Autodesk Fusion 360 part; units mm, degrees
sketch "草图1" plane through (0, 0, 0) normal (0, 0, 1) x (1, 0, 0)
  line L0 (28.4627, -32.3648) -> (28.4702, -32.3737)
  line L1 (41.5939, -11.2943) -> (41.768, -11.325)
  arc A0 (14.7507, -46.3074) -> (13.8402, -43.4489) centre (14.2954, -44.8782) ccw construction
  line L2 (-28.4627, -32.3648) -> (-28.4702, -32.3737)
  circle A1 centre (0, -47.1) radius 1.4
  line L3 (43.1, 0) -> (48, 0) construction
  line L4 (0, -43.1) -> (0, -51.1) construction
  arc A2 (2.5554, -45.5283) -> (2.6381, -48.5283) centre (0, -47.1) ccw construction
  circle A3 centre (0, 0) radius 44.72 construction
  arc A4 (2.6381, -48.5283) -> (14.7507, -46.3074) centre (0, 0) ccw construction
  line L5 (-30.5781, -30.3742) -> (-30.6917, -30.5096)
  line L6 (-41.5939, -11.2943) -> (-41.768, -11.325)
  line L7 (30.5781, -30.3742) -> (30.6917, -30.5096)
  line L8 (42.2601, -8.467) -> (42.2716, -8.469)
  line L9 (-42.2601, -8.467) -> (-42.2716, -8.469)
  line L10 (0.9, -43.0906) -> (0.9, -43.1)
  arc A5 (2.5554, -45.5283) -> (13.8402, -43.4489) centre (0, 0) ccw construction
  line L11 (-0.9, -43.0906) -> (-0.9, -43.1)
  circle A6 centre (0, 0) radius 43.1
  arc A7 (40.7077, 26.5489) -> (32.728, 35.9282) centre (0, 0) ccw construction
  line L12 (11.0158, 41.6685) -> (11.0763, 41.8346)
  line L13 (13.7974, 40.8319) -> (13.8014, 40.8428)
  line L14 (36.8676, 22.3247) -> (36.8757, 22.3294)
  arc A8 (32.728, 35.9282) -> (30.7078, 33.7104) centre (31.7179, 34.8193) ccw construction
  circle A9 centre (40.7898, 23.55) radius 1.4
  circle A10 centre (-40.7898, 23.55) radius 1.4
  line L15 (-15.6751, 9.05) -> (-16.3679, 9.45) construction
  arc A11 (38.151, 24.9772) -> (30.7078, 33.7104) centre (0, 0) ccw construction
  line L16 (-13.7974, 40.8319) -> (-13.8014, 40.8428)
  line L17 (37.7676, 20.7659) -> (37.7757, 20.7706)
  arc A12 (-40.7064, 20.5512) -> (-44.548, 9.7385) centre (0, 0) ccw construction
  arc A13 (-47.4788, 10.3792) -> (-44.548, 9.7385) centre (-46.0134, 10.0589) ccw construction
  circle A14 centre (0, 0) radius 47.1 construction
  arc A15 (-43.3459, 21.9795) -> (-47.4788, 10.3792) centre (0, 0) ccw construction
  line L18 (-37.7676, 20.7659) -> (-37.7757, 20.7706)
  line L19 (-36.8676, 22.3247) -> (-36.8757, 22.3294)
  arc A16 (38.151, 24.9772) -> (40.7077, 26.5489) centre (40.7898, 23.55) ccw construction
  circle A17 centre (0, 0) radius 47.1 construction
  line L20 (-11.0158, 41.6685) -> (-11.0763, 41.8346)
  line L21 (-37.3257, 21.55) -> (-41.5692, 24) construction
  arc A18 (-40.7064, 20.5512) -> (-43.3459, 21.9795) centre (-40.7898, 23.55) ccw construction
  circle A19 centre (0, 0) radius 46.9
  arc A20 (32.5934, 35.7803) -> (30.8425, 33.8583) centre (31.7179, 34.8193) ccw
  arc A21 (38.3851, 24.9844) -> (30.8425, 33.8583) centre (0, 0) ccw
  arc A22 (38.3851, 24.9844) -> (40.6026, 26.3437) centre (40.7898, 23.55) ccw
  arc A23 (40.6026, 26.3437) -> (32.5934, 35.7803) centre (0, 0) ccw
  arc A24 (2.4446, -45.7347) -> (13.9009, -43.6395) centre (0, 0) ccw
  arc A25 (14.69, -46.1168) -> (13.9009, -43.6395) centre (14.2954, -44.8782) ccw
  arc A26 (2.5131, -48.3347) -> (14.69, -46.1168) centre (0, 0) ccw
  arc A27 (2.4446, -45.7347) -> (2.5131, -48.3347) centre (0, -47.1) ccw
  arc A28 (-47.2834, 10.3365) -> (-44.7434, 9.7812) centre (-46.0134, 10.0589) ccw
  arc A29 (-40.8297, 20.7503) -> (-44.7434, 9.7812) centre (0, 0) ccw
  arc A30 (-40.8297, 20.7503) -> (-43.1156, 21.991) centre (-40.7898, 23.55) ccw
  arc A31 (-43.1156, 21.991) -> (-47.2834, 10.3365) centre (0, 0) ccw
  circle A32 centre (0, 0) radius 19.5
  dimension "d43" = 1.8
  dimension "d44" = 6
  dimension "d45" = 3
  dimension "d46" = 2.8
  dimension "d47" = 2.8
  dimension "d48" = 2.8
  dimension "d49" = 86.2
  dimension "d53" = -0.2
  dimension "d54" = -0.2
  dimension "d55" = -0.2
  dimension "d56" = -0.2
  dimension "d57" = 39
extrude "拉伸5" add sketch "草图1" along normal blind 1.8 contours A1 A19 A25 A26 A27 | A1 A19 A24 A25 A27 | A19 A20 A21 A22 A24 A25 A27 A28 A29 A30 | A10 A19 A28 A30 A31 | A10 A19 A28 A29 A30 | A9 A19 A20 A21 A22 | A9 A19 A20 A22 A23
extrude "拉伸6" add sketch "草图1" along normal up to surface (1.8 mm away) contours A6
sketch "草图3" plane through (0, 0, 1.8) normal (0, 0, 1) x (-1, 0, 0)
  circle A0 centre (0, 0) radius 19.5
  circle A1 centre (40.7898, -23.55) radius 1.4
  circle A2 centre (-40.7898, -23.55) radius 1.4
  circle A3 centre (0, 47.1) radius 1.4
  arc A4 (43.1156, -21.991) -> (47.2834, -10.3365) centre (0, 0) ccw
  arc A5 (47.2834, -10.3365) -> (46.0746, -8.7603) centre (46.0134, -10.0589) ccw
  arc A6 (46.0746, -8.7603) -> (2.7857, 46.8172) centre (0, 0) ccw
  arc A7 (2.7857, 46.8172) -> (-2.5131, 48.3347) centre (0, 47.1) ccw
  arc A8 (-2.5131, 48.3347) -> (-14.69, 46.1168) centre (0, 0) ccw
  arc A9 (-14.69, 46.1168) -> (-15.4506, 44.2819) centre (-14.2954, 44.8782) ccw
  arc A10 (-15.4506, 44.2819) -> (-41.9377, -20.9961) centre (0, 0) ccw
  arc A11 (-41.9377, -20.9961) -> (-40.6026, -26.3437) centre (-40.7898, -23.55) ccw
  arc A12 (-40.6026, -26.3437) -> (-32.5934, -35.7803) centre (0, 0) ccw
  arc A13 (-32.5934, -35.7803) -> (-30.6239, -35.5216) centre (-31.7179, -34.8193) ccw
  arc A14 (-30.6239, -35.5216) -> (39.152, -25.8211) centre (0, 0) ccw
  arc A15 (39.152, -25.8211) -> (43.1156, -21.991) centre (40.7898, -23.55) ccw
  circle A16 centre (0, 0) radius 29.75
  dimension "d64" = 59.5
sketch "草图4" plane through (0, 0, 0) normal (0, 0, -1) x (1, 0, 0)
  circle A0 centre (0, 0) radius 19.5
  circle A1 centre (-40.7898, -23.55) radius 1.4
  circle A2 centre (40.7898, -23.55) radius 1.4
  circle A3 centre (0, 47.1) radius 1.4
  arc A4 (-47.2834, -10.3365) -> (-43.1156, -21.991) centre (0, 0) ccw
  arc A5 (-43.1156, -21.991) -> (-39.152, -25.8211) centre (-40.7898, -23.55) ccw
  arc A6 (-39.152, -25.8211) -> (30.6239, -35.5216) centre (0, 0) ccw
  arc A7 (30.6239, -35.5216) -> (32.5934, -35.7803) centre (31.7179, -34.8193) ccw
  arc A8 (32.5934, -35.7803) -> (40.6026, -26.3437) centre (0, 0) ccw
  arc A9 (40.6026, -26.3437) -> (41.9377, -20.9961) centre (40.7898, -23.55) ccw
  arc A10 (41.9377, -20.9961) -> (15.4506, 44.2819) centre (0, 0) ccw
  arc A11 (15.4506, 44.2819) -> (14.69, 46.1168) centre (14.2954, 44.8782) ccw
  arc A12 (14.69, 46.1168) -> (2.5131, 48.3347) centre (0, 0) ccw
  arc A13 (2.5131, 48.3347) -> (-2.7857, 46.8172) centre (0, 47.1) ccw
  arc A14 (-2.7857, 46.8172) -> (-46.0746, -8.7603) centre (0, 0) ccw
  arc A15 (-46.0746, -8.7603) -> (-47.2834, -10.3365) centre (-46.0134, -10.0589) ccw
  circle A16 centre (0, 0) radius 43.1
  dimension "d65" = 86.2
extrude "拉伸8" add sketch "草图4" along normal blind 18 contours A16
extrude "拉伸9" cut sketch "草图3" against normal blind 5.5 contours A16
sketch "草图5" plane through (0, 0, -3.7) normal (0, 0, 1) x (-1, 0, 0)
  circle A0 centre (0, 0) radius 19.5
  circle A1 centre (0, 0) radius 29.75
  line L0 (0.0358, 19.5) -> (0.0358, 29.75)
  line L1 (8.0358, 17.7673) -> (8.0358, 28.6442)
  line L2 (-7.9642, 17.7673) -> (-7.9642, 28.6642)
extrude "拉伸10" cut sketch "草图5" against normal blind 20 contours A0 A1 L0 L1 | A0 A1 L0 L2
sketch "草图6" plane through (0, 0, -18) normal (0, 0, -1) x (1, 0, 0)
  circle A0 centre (0, 0) radius 43.1
  line L0 (-8.0358, 17.7673) -> (-8.0358, 28.6442)
  arc A1 (7.9642, 28.6642) -> (-8.0358, 28.6442) centre (0, 0) ccw
  line L1 (7.9642, 28.6642) -> (7.9642, 17.7995)
  arc A2 (-8.0358, 17.7673) -> (7.9642, 17.7995) centre (0, 0) ccw
  circle A3 centre (0, 0) radius 35
  circle A4 centre (0, -35) radius 1.31
  circle A5 centre (35, 0) radius 1.31
  circle A6 centre (0, 35) radius 1.31
  circle A7 centre (-35, 0) radius 1.31
  dimension "d73" = 70
  dimension "d74" = 2.62
  dimension "d76" = 360
extrude "拉伸11" cut sketch "草图6" against normal blind 8 contours A3 A5 | A3 A5 | A3 A6 | A3 A6 | A3 A4 | A3 A4 | A3 A7 | A3 A7
sketch "草图7" plane through (0, 0, -18) normal (0, 0, -1) x (1, 0, 0)
  circle A0 centre (35, 0) radius 1.31
  circle A1 centre (-35, 0) radius 1.31
  circle A2 centre (0, -35) radius 1.31
  circle A3 centre (0, 35) radius 1.31
  circle A4 centre (0, 0) radius 43.1
  line L0 (-8.0358, 17.7673) -> (-8.0358, 28.6442)
  arc A5 (7.9642, 28.6642) -> (-8.0358, 28.6442) centre (0, 0) ccw
  line L1 (7.9642, 28.6642) -> (7.9642, 17.7995)
  arc A6 (-8.0358, 17.7673) -> (7.9642, 17.7995) centre (0, 0) ccw
  circle A7 centre (0, 0) radius 30
  dimension "d79" = 60
extrude "拉伸12" cut sketch "草图7" against normal blind 10 contours A7
extrude "拉伸13" add 1 faces at (34.9911, 7.617, -18) along direction (0, 0, -1) blind 6
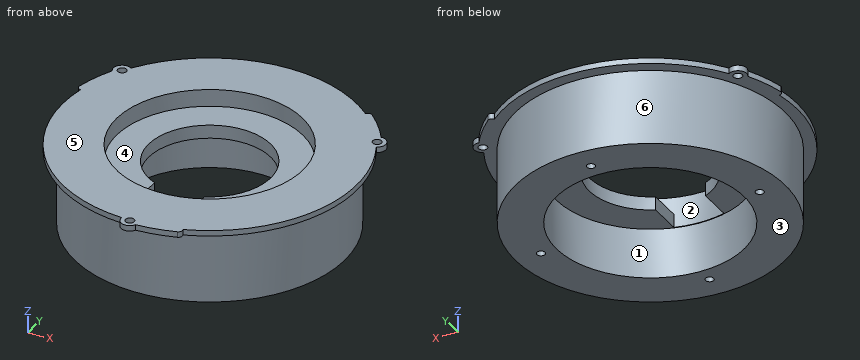
Here's how the part is built. I have some questions about the finished solid (model axes, mm). Face numbers are marked on the shaded views. A direction names the side the tool comes from. Give positions to 0.01 mm unless a question says otherwise; leave off trailing zeros. Order: outer loops, then holes, each group sorted by start corner. A loop starts at its lowest first (then second) coordinate and runs counter-clockwise, first axis right, second up. Notation, with made-up numbers: M 2.25,48 L 15.25,48 A26 ccw 15.25,62 Z; hole C -25,11.25 d9. An arc over 180 degrees is marked long. Use a Markdown table: item, result. Add a question column.
1. Suppose I cut it at A-A (x = 0). Give the number of separate pieces and of enclosed holes in the cut face, and give its area (3 significant figures).
2. For pin 1 Ø3 at (x, z) = (20.5, -2) entering from -Y; pin 2 Ø2 at (x, z) = (-25, -17) entering from -Y; pin 3 Ø4 at (x, z) = (-15, -16.5) entering from -Y, each with a flat end and sliding along its axis, tell me the tip position at first contact or that it passes through.
3. If we mould it in two halves opening along X, with no side actions, what happens to the marked faces 4, 5 and 6? For each: +X half, -X half, draft (parallel to the pull), parting line (faces both ways), or undercut.
4. Suppose I cut it at D-D (y = 23.55). List the corners of the cut face in (x, z) for me.
5. Suppose I cut it at C-C (z = -14.75). List the corners of the cut face in (x, y) for me, and give its area (3 significant figures).
6. I need wall thicknesses on probe 1 along X at (y, z) = (0, -5); probe 2 along X at (y, z) = (0, -14.5); probe 3 along Y at (x, z) = (0.5, -0.5). Which ranges of each line are inside material? Lowest first, please. Write a range as from..to.
7. Suppose I cut it at B-B (y = 0). List the corners of the cut face in (x, z) for me, and give its area (3 significant figures).
8. On a 3-axis mill with a long thin cutter (end or side, diameter ignored), from which of +Z, -Z, +X, -X, +Y, -Y can I reach the whole of each face in a straight line? I mean the marked faces 1, 2 and 3. Say none if no direction works.
Results list:
| question | item | result |
|---|---|---|
| 1 | separate pieces | 3 |
| 1 | enclosed holes | 0 |
| 1 | area | 666 mm² |
| 2 | pin 1 | stops at y = -38.69 |
| 2 | pin 2 | stops at y = -35.8 |
| 2 | pin 3 | stops at y = -41.09 |
| 3 | face 4 | undercut |
| 3 | face 5 | draft |
| 3 | face 6 | parting line |
| 4 | outline | M -43.59,0 L -42.19,0 L -42.19,1.8 L -43.59,1.8 Z; M -39.39,0 L -36.1,0 L -36.1,-24 L -18.58,-24 L -18.58,-8 L 18.58,-8 L 18.58,-24 L 36.1,-24 L 36.1,0 L 39.39,0 L 39.39,1.8 L 18.18,1.8 L 18.18,-3.7 L -18.18,-3.7 L -18.18,1.8 L -39.39,1.8 Z; M 42.19,0 L 43.59,0 L 43.59,1.8 L 42.19,1.8 Z |
| 5 | outline | C 0,0 d86.2; hole C -35,0 d2.62; hole C 0,0 d60; hole C 0,-35 d2.62; hole C 0,35 d2.62; hole C 35,0 d2.62 |
| 5 | area | 2,990 mm² |
| 6 | probe 1 | x = -43.1..-19.5, 19.5..43.1 |
| 6 | probe 2 | x = -43.1..-36.31, -33.69..-30, 30..33.69, 36.31..43.1 |
| 6 | probe 3 | y = -43.1..-29.75, 29.75..43.1 |
| 7 | outline | M -46.9,0 L -43.1,0 L -43.1,-24 L -36.31,-24 L -36.31,-10 L -33.69,-10 L -33.69,-24 L -30,-24 L -30,-8 L -19.5,-8 L -19.5,-3.7 L -29.75,-3.7 L -29.75,1.8 L -46.9,1.8 Z; M 19.5,-8 L 30,-8 L 30,-24 L 33.69,-24 L 33.69,-10 L 36.31,-10 L 36.31,-24 L 43.1,-24 L 43.1,0 L 46.9,0 L 46.9,1.8 L 29.75,1.8 L 29.75,-3.7 L 19.5,-3.7 Z |
| 7 | area | 709 mm² |
| 8 | face 1 | -Z |
| 8 | face 2 | +Z |
| 8 | face 3 | -Z, +X, -X, +Y, -Y |
